Here's how the part is built. I have some questions about the finished solid (model axes, mm). A direction names the side the tool comes from. Coordinates: 2 decimals unless noted, no trailing zeros. Write each loop counter-clockwise with the first axis right and the second up, starting at its lowest first coordinate (ties: lowest second). Pieces come first, ordered by that corner, then holes.
Autodesk Inventor part; units mm, degrees
ref_plane "YZ Plane" through (0, 0, 0) normal (1, 0, 0) x (0, 1, 0)
ref_plane "XZ Plane" through (0, 0, 0) normal (0, 1, 0) x (-1, 0, 0)
ref_plane "XY Plane" through (0, 0, 0) normal (0, 0, 1) x (1, 0, 0)
sketch "Sketch1" plane through (0, 0, 0) normal (0, 0, 1) x (1, 0, 0)
  line L0 (76.2, -12.7) -> (-76.2, -12.7)
  line L1 (-76.2, -12.7) -> (-76.2, 12.7)
  line L2 (-76.2, 12.7) -> (76.2, 12.7)
  line L3 (76.2, 12.7) -> (76.2, -12.7)
  line L4 (76.2, -12.7) -> (-76.2, 12.7) construction
  line L5 (-76.2, -12.7) -> (76.2, 12.7) construction
  line L6 (-76.2, 12.7) -> (-72.39, 12.7)
  line L7 (-72.39, 12.7) -> (-72.39, -12.7)
  line L8 (-72.39, -12.7) -> (-76.2, -12.7)
  line L9 (-76.2, -12.7) -> (-76.2, 12.7)
  line L10 (76.2, 12.7) -> (72.39, 12.7)
  line L11 (72.39, 12.7) -> (72.39, -12.7)
  line L12 (72.39, -12.7) -> (76.2, -12.7)
  line L13 (76.2, -12.7) -> (76.2, 12.7)
  point P0 (0, 0)
  dimension "d0" = 152.4
  dimension "d1" = 25.4
  dimension "d2" = 3.81
  dimension "d3" = 3.81
extrude "Extrusion1" add sketch "Sketch1" along normal blind 3.175 contours L0 L7 L2 L11
extrude "Extrusion2" add sketch "Sketch1" along normal blind 41.275 contours L0 L11 L2 L3 | L0 L1 L2 L7
chamfer "Chamfer1" distance 3.175 angle 45 2 edges at (-76.2, 0, 41.275) (76.2, 0, 41.275)
sketch "Sketch2" plane through (76.2, -12.7, 0) normal (1, 0, 0) x (0, 0, -1)
  line L0 (-3.175, 25.4) -> (-41.275, 25.4) construction
  line L1 (-22.225, 25.4) -> (-22.225, 0) construction
  line L2 (0, 0) -> (-38.1, 0) construction
  line L3 (-41.275, 0) -> (-41.275, 25.4) construction
  line L4 (-41.275, 12.7) -> (0, 12.7) construction
  circle A0 centre (-22.225, 12.7) radius 2.25
  line L5 (-3.175, 0) -> (-3.175, 25.4)
  dimension "d11" = 4.5
  dimension "d14" = 19.05
extrude "Extrusion3" cut sketch "Sketch2" against normal through all
properties part number "New_Arm_Brace"
1) On a 3-axis mill with a long thin cutter (end or side, diameter ignored), from which of +Z, -Z, +X, -X, +Y, -Y can I reach the whole of each face in a straight line? I mean faces 1 (the face through (-72.39, -3, 22)), 2 (the face through (-1, 0, 0)). Say none if no direction works.
Values follow:
face 1: +Z, +Y, -Y
face 2: -Z, +X, -X, +Y, -Y
2) Imagine slicing it at B-B on y = -5.5. Please give me the cut outline in (x, z) (3 decimals), then the cut area to 3 significant figures.
Values follow:
outline: (-76.2, 0) - (76.2, 0) - (76.2, 38.1) - (73.025, 41.275) - (72.39, 41.275) - (72.39, 3.175) - (-72.39, 3.175) - (-72.39, 41.275) - (-73.025, 41.275) - (-76.2, 38.1) - close
area: 764 mm2
3) Will these pins go through, and if not, where does the flat tip stop? pin 1 (2 mm diameter, centred on x = -5, y = 10, fed in from +Z) (3 decimals); pin 2 (8 mm diameter, centred on x = -27.5, y = 3.5, fed in from -Z).
Values follow:
pin 1: stops at z = 3.175
pin 2: stops at z = 0
4) I need wall thicknesses on probe 1 along X at (y, z) = (-2.25, 27); probe 2 along Z at (x, y) = (3.5, -9) (3 decimals); probe 3 along X at (y, z) = (-2.25, 39.5). Which ranges of each line are inside material? Lowest first, please.
Values follow:
probe 1: x = -76.2 to -72.39, 72.39 to 76.2
probe 2: z = 0 to 3.175
probe 3: x = -74.8 to -72.39, 72.39 to 74.8
5) Imagine slicing it at C-C on x = -36. Please give me the cut outline in (y, z) (3 decimals), then the cut area to 3 significant figures.
Values follow:
outline: (-12.7, 0) - (12.7, 0) - (12.7, 3.175) - (-12.7, 3.175) - close
area: 80.6 mm2
6) Imagine slicing it at A-A on z = 22. Please give me the cut outline in (x, y).
Values follow:
outline: (-76.2, -12.7) - (-72.39, -12.7) - (-72.39, -2.24) - (-76.2, -2.24) - close; (-76.2, 2.24) - (-72.39, 2.24) - (-72.39, 12.7) - (-76.2, 12.7) - close; (72.39, -12.7) - (76.2, -12.7) - (76.2, -2.24) - (72.39, -2.24) - close; (72.39, 2.24) - (76.2, 2.24) - (76.2, 12.7) - (72.39, 12.7) - close
7) We'd pull the mould along X, two halves only. Please class faces 3 (the face through (-1, 0, 3.175)), 4 (the face through (74.32, 0.68, 20.08)), 5 (the face through (72.39, -3, 22)), 6 (the face through (-74.6, 0.2, 39.7)): pulls with the +X half, pulls with the -X half, needs draft (parallel to the pull), parting line crosses it, or undercut.
Values follow:
face 3: undercut
face 4: needs draft
face 5: undercut
face 6: pulls with the -X half
